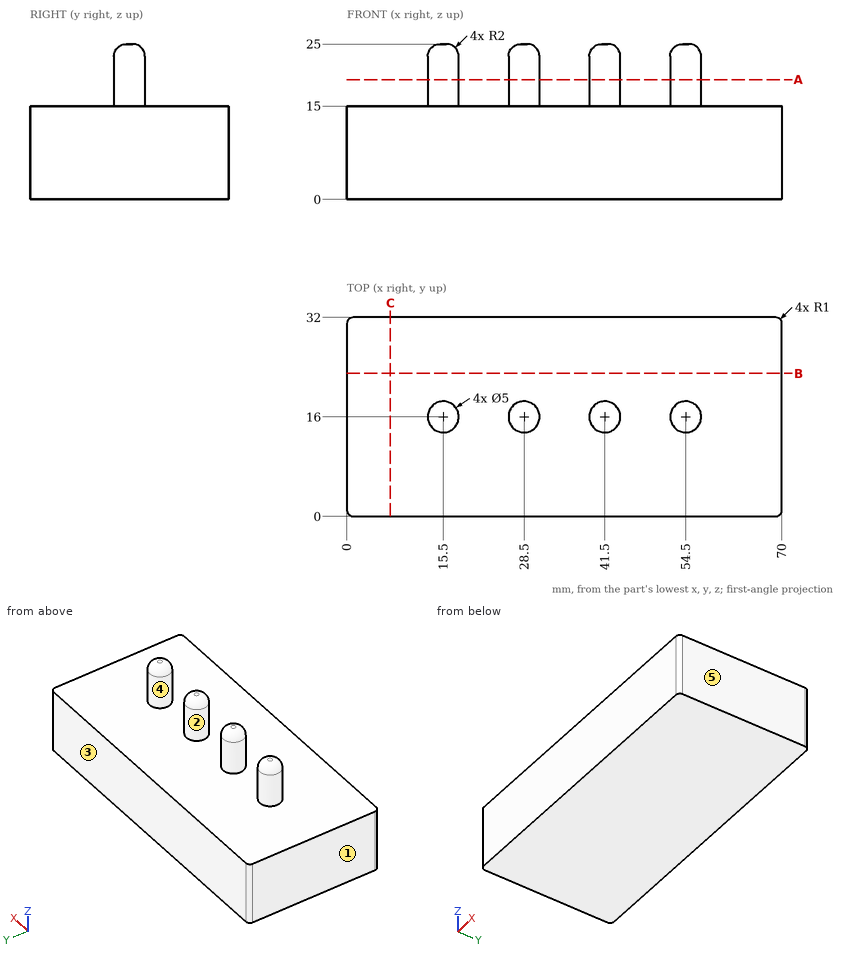
Can you work these out from the drawing? Everything is in mm from the part's minimum corner. A direction names the side the tool comes from. Coordinates: 2 decimals unless noted, no trailing zeros. Write each loop counter-clockwise with the first axis right and the second up, starting at its lowest first coordinate (ties: lowest second). Pieces come first, ordered by that corner, then holes. Notation, with made-up numbers: (71, 3.5) -> (109, 3.5) arc R12 ccw to (109, 22.5) -> close; hole circle Ø11 at (79.5, 12.5). An arc over 180 degrees is marked (long way). Write item = value, one per line.
(1) Imagine slicing it at B-B (y = 23). Please give me the cut outline in (x, z).
Verdict:
outline = (0, 0) -> (70, 0) -> (70, 15) -> (0, 15) -> close
(2) For pin 1 (2 mm diameter, centred on x = 37, y = 7, fed in from +Z); pin 2 (6 mm diameter, centred on x = 38, z = 19.5, fed in from +Y), each with a flat end and sliding along its axis, tell me the tip position at first contact or that it passes through.
Verdict:
pin_1 = 15
pin_2 = 18.45
(3) Imagine slicing it at A-A (z = 19.25). Please give me the cut outline in (x, y), and give its area (3 significant figures).
Verdict:
outline = circle Ø5 at (15.5, 16); circle Ø5 at (28.5, 16); circle Ø5 at (41.5, 16); circle Ø5 at (54.5, 16)
area = 78.5 mm^2
(4) On a 3-axis mill with a long thin cutter (end or side, diameter ignored), from which of +Z, -Z, +X, -X, +Y, -Y can I reach the whole of each face in a straight line? I mean the marked faces 4 and 5. Say none if no direction works.
Verdict:
face_4 = +Z
face_5 = +Z, -Z, +X, +Y, -Y
(5) Thinking about a two-plate mould opening in X: for the marked faces 1, 2 and 3, which applies, +X half, -X half, draft (parallel to the pull), parting line (faces both ways), or undercut?
Verdict:
face_1 = -X half
face_2 = undercut
face_3 = draft
(6) If I drill on probe 1 along X at (y, z) = (18, 16); probe 2 along Z at (x, y) = (54, 26); probe 3 along Y at (x, z) = (56, 22.5), over which ranges is the centre line in solid material (lowest first)?
Verdict:
probe_1 = 14 to 17, 27 to 30, 40 to 43, 53 to 56
probe_2 = 0 to 15
probe_3 = 14 to 18
(7) Imagine slicing it at C-C (x = 7). Please give me the cut outline in (y, z).
Verdict:
outline = (0, 0) -> (32, 0) -> (32, 15) -> (0, 15) -> close
